```python
from build123d import *

# Parameters (mm, degrees)
SKETCH2_W      = 587
SKETCH2_H      = 303
BASE_DEPTH     = 10
SKETCH4_W      = 587
SKETCH4_H      = 303
SKETCH4_W_2    = 567
SKETCH4_H_2    = 283
WALLS_DEPTH    = 380
LID_DEPTH      = 10
LID_DEPTH_BACK = 597
SKETCH5_W      = 323
SKETCH5_H      = 10
INLET_REACH    = 529.441
SKETCH8_R      = 10
OUTLET_REACH   = 529.441
SKETCH9_R      = 10


with BuildPart() as part:
    # Sketch2 → Base (new body)
    with BuildSketch(Plane(origin=(0, 0, 0), x_dir=(1, 0, 0), z_dir=(0, 1, 0))):
        Rectangle(SKETCH2_W, SKETCH2_H)
    extrude(amount=BASE_DEPTH)

    # Sketch4 → Walls (add)
    with BuildSketch(Plane(origin=(0, 10, 0), x_dir=(1, 0, 0), z_dir=(0, 1, 0))):
        Rectangle(SKETCH4_W, SKETCH4_H)
        Rectangle(SKETCH4_W_2, SKETCH4_H_2, mode=Mode.SUBTRACT)
    extrude(amount=WALLS_DEPTH)

    # Sketch5 → Lid (add, two sides: drawn at the far end of the back side and taken through both)
    with BuildSketch(Plane.ZY.offset(293.5).offset(-LID_DEPTH_BACK)):
        with Locations((0, 395)):
            Rectangle(SKETCH5_W, SKETCH5_H)
    extrude(amount=LID_DEPTH + LID_DEPTH_BACK)

    # Sketch8 → Inlet (cut, up to next)
    with BuildSketch(Plane(origin=(0, 400, 0), x_dir=(1, 0, 0), z_dir=(0, 1, 0)), mode=Mode.PRIVATE) as inlet_sk1:
        with Locations(Location((0, 0, 0), (0, 0, 270))):
            Circle(SKETCH8_R)
    inlet_tool1 = extrude(inlet_sk1.sketch, amount=-INLET_REACH, mode=Mode.PRIVATE) & part.part
    add(inlet_tool1.solids().sort_by_distance((0, 400, 0))[0], mode=Mode.SUBTRACT)

    # Sketch9 → Outlet (cut, up to next)
    with BuildSketch(Plane.XZ, mode=Mode.PRIVATE) as outlet_sk1:
        with Locations(Location((-248.5, 0, 0), (0, 0, 270))):
            Circle(SKETCH9_R)
    outlet_tool1 = extrude(outlet_sk1.sketch, amount=-OUTLET_REACH, mode=Mode.PRIVATE) & part.part
    add(outlet_tool1.solids().sort_by_distance((-248.5, 0, 0))[0], mode=Mode.SUBTRACT)


solid = part.part
```
CAD build for the part. Positions are in the model's coordinates, mm. A direction names the side the tool comes from. Round coordinates to 2 decimals unless told otherwise and drop trailing zeros. Order: outer loops, then holes, each group sorted by start corner. A loop starts at its lowest first (then second) coordinate and runs counter-clockwise, first axis right, second up.
Q1. Which spindle directions (+Z, -Z, +X, -X, +Y, -Y) get a long thin tool onto all of the face, cutting with end or side? Do faces 1 (the flat face through (-293.5, 192, 2)), 2 (the cylindrical face through (-257.372, 4.93, -4.614)), 3 (the flat face through (-283.5, 197, 2)), 4 (the flat face through (-4, 192, 151.5)), 5 (the cylindrical face through (-9.76, 395.07, -2.17)). Say none if no direction does.
Q2. Slice it at D-D (x = -52.5). Write the cut outline in (y, z), and give its area (3 significant figures).
Q3. Slice it at A-A (z = -67.5). Write the cut outline in (x, y).
Q4. Wall check: L1, parallel to Z at x = 150, y = 280.5; L2, parallel to Y at x = -67.5, z = -11; L3, parallel to X at y = 392, z = 0. Give the ranges that are in metal, low to high.
Q5. Two-plate mould, pull along Z, no slides. Class faces 6 (the flat face through (293.5, 192, 2)), 7 (the flat face through (-4, 197, 141.5)), 8 (the flat face through (-4, 192, -151.5)): pulls with the +Z half, pulls with the -Z half, needs draft (parallel to the pull), parting line crosses it, or undercut.
Q6. Drop flat-ended pins along their axis: pin 1 (2 mm diameter, centred on x = -89.5, z = 56, fed in from -Y); pin 2 (5 mm diameter, centred on x = -20.5, y = 60, fed in from +Z); pin 3 (2 mm diameter, centred on y = 201, z = 29.5, fed in from -X); pin 4 (3 mm diameter, centred on y = 313, z = 22, fed in from +X). Give the stop position or say it passes through.
Q7. Slice it at C-C (z = 0). Write the cut outline in (x, y).
Q8. Slice it at B-B (y = 355). Write the cut outline in (x, z), and give its area (3 significant figures).
Results below:
1. face 1: +Z, -Z, -X, -Y
1. face 2: -Y
1. face 3: none
1. face 4: +Z, +X, -X, -Y
1. face 5: +Y
2. outline: (0, -151.5) - (390, -151.5) - (390, -161.5) - (400, -161.5) - (400, 161.5) - (390, 161.5) - (390, 151.5) - (0, 151.5) - close; hole (10, -141.5) - (390, -141.5) - (390, 141.5) - (10, 141.5) - close
2. area: 13,900 mm2
3. outline: (-303.5, 390) - (-293.5, 390) - (-293.5, 0) - (293.5, 0) - (293.5, 390) - (303.5, 390) - (303.5, 400) - (-303.5, 400) - close; hole (-283.5, 10) - (283.5, 10) - (283.5, 390) - (-283.5, 390) - close
4. L1: z = -151.5 to -141.5, 141.5 to 151.5
4. L2: y = 0 to 10, 390 to 400
4. L3: x = -303.5 to -10, 10 to 303.5
5. face 6: needs draft
5. face 7: undercut
5. face 8: pulls with the -Z half
6. pin 1: stops at y = 0
6. pin 2: stops at z = 151.5
6. pin 3: stops at x = -293.5
6. pin 4: stops at x = 293.5
7. outline: (-303.5, 390) - (-293.5, 390) - (-293.5, 0) - (-258.5, 0) - (-258.5, 10) - (-283.5, 10) - (-283.5, 390) - (-10, 390) - (-10, 400) - (-303.5, 400) - close; (-238.5, 0) - (293.5, 0) - (293.5, 390) - (303.5, 390) - (303.5, 400) - (10, 400) - (10, 390) - (283.5, 390) - (283.5, 10) - (-238.5, 10) - close
8. outline: (-293.5, -151.5) - (293.5, -151.5) - (293.5, 151.5) - (-293.5, 151.5) - close; hole (-283.5, -141.5) - (283.5, -141.5) - (283.5, 141.5) - (-283.5, 141.5) - close
8. area: 17,400 mm2
